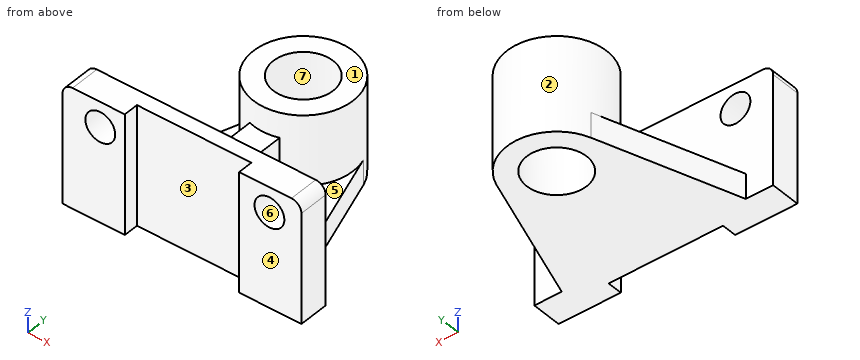
Autodesk Inventor part; units mm, degrees
ref_plane "YZ Plane" through (0, 0, 0) normal (1, 0, 0) x (0, 1, 0)
ref_plane "XZ Plane" through (0, 0, 0) normal (0, 1, 0) x (-1, 0, 0)
ref_plane "XY Plane" through (0, 0, 0) normal (0, 0, 1) x (1, 0, 0)
sketch "草图1" plane through (0, 0, 0) normal (0, 1, 0) x (-1, 0, 0)
  line L0 (24, 0) -> (-24, 0)
  line L1 (-24, 0) -> (-24, 22)
  line L2 (-22, 24) -> (22, 24)
  line L3 (24, 22) -> (24, 0)
  line L4 (0, 29.295577) -> (0, -8.008859)
  arc A0 (24, 22) -> (22, 24) centre (22, 22) ccw
  arc A1 (-22, 24) -> (-24, 22) centre (-22, 22) ccw
  line L5 (28.197943, 19) -> (-37.870085, 19) construction
  circle A2 centre (16.428853, 19) radius 3
  circle A3 centre (-17.571147, 19) radius 3
  point P0 (0, 0)
  point P1 (-24, 24)
  dimension "d0" = 24
  dimension "d1" = 48
  dimension "d2" = 2
  dimension "d3" = 5
  dimension "d4" = 6
  dimension "d5" = 6
  dimension "d6" = 34
extrude "拉伸1" add sketch "草图1" along normal blind 6
sketch "草图2" plane through (0, 0, 0) normal (0, 0, 1) x (1, 0, 0)
  line L0 (22, 0) -> (-22, 0)
  line L1 (22, 0) -> (22, 6)
  line L2 (-22, 6) -> (22, 6)
  line L3 (-22, 0) -> (-22, 6)
  line L4 (11.5, -3) -> (-11.5, -3)
  line L5 (-11.5, -3) -> (-11.5, 3)
  line L6 (-11.5, 3) -> (11.5, 3)
  line L7 (11.5, 3) -> (11.5, -3)
  line L8 (11.5, -3) -> (-11.5, 3) construction
  line L9 (-11.5, -3) -> (11.5, 3) construction
  point P0 (0, 0)
  dimension "d9" = 23
  dimension "d10" = 6
extrude "拉伸2" cut sketch "草图2" along normal blind 30 contours L7 L4 L5 L0 | L0 L5 L6 L7
sketch "草图3" plane through (0, 0, 0) normal (0, 0, 1) x (1, 0, 0)
  circle A0 centre (0, 30) radius 10
  line L0 (11.5, 3) -> (11.5, 0)
  line L1 (22, 0) -> (11.5, 0)
  line L2 (22, 0) -> (22, 6)
  line L3 (-22, 6) -> (22, 6)
  line L4 (-22, 0) -> (-22, 6)
  line L5 (-11.5, 0) -> (-22, 0)
  line L6 (-11.5, 0) -> (-11.5, 3)
  line L7 (-11.5, 3) -> (11.5, 3)
  line L8 (0, -6.997144) -> (0, 46.686565)
  circle A1 centre (0, 30) radius 6
  point P0 (0, 0)
  dimension "d13" = 20
  dimension "d14" = 30
  dimension "d15" = 12
extrude "拉伸3" add sketch "草图3" along normal blind 19 contours A0 L8 A1 | L8 A1 A0
sketch "草图4" plane through (0, 30, 0) normal (0, 0, -1) x (-1, 0, 0)
  circle A0 centre (0, 0) radius 10
  line L0 (-11.5, -30) -> (-11.5, -27)
  line L1 (-11.5, -27) -> (11.5, -27)
  line L2 (11.5, -27) -> (11.5, -30)
  line L3 (24, -30) -> (11.5, -30)
  line L4 (24, -30) -> (24, -24)
  line L5 (-24, -24) -> (24, -24)
  line L6 (-24, -30) -> (-24, -24)
  line L7 (-11.5, -30) -> (-24, -30)
  line L8 (-9.4744, 3.199335) -> (-18.5, -24)
  line L9 (9.4744, 3.199335) -> (18.5, -24)
  line L10 (0, -31.113393) -> (0, 9.909735)
  point P0 (0, -30)
  dimension "d18" = 37
sketch "草图4 outline for 拉伸4" plane through (0, 30, 0) normal (0, 0, -1) x (-1, 0, 0)
  line L0 (18.5, -24) -> (9.4744, 3.199335)
  line L1 (-18.5, -24) -> (18.5, -24)
  line L2 (-9.4744, 3.199335) -> (-18.5, -24)
  arc A0 (-9.4744, 3.199335) -> (9.4744, 3.199335) centre (0, 0) ccw
extrude "拉伸4" add sketch "草图4 outline for 拉伸4" against normal blind 5
sketch "草图5" plane through (0, 30, 5) normal (0, 0, 1) x (1, 0, 0)
  arc A0 (-9.507538, 3.099472) -> (9.507538, 3.099472) centre (0, 0) ccw
  line L0 (18.5, -24) -> (-18.5, -24)
  line L1 (3, -8) -> (-3, -8)
  line L2 (-3, -8) -> (-3, -24)
  line L3 (-3, -24) -> (3, -24)
  line L4 (3, -24) -> (3, -8)
  line L5 (3, -8) -> (-3, -24) construction
  line L6 (-3, -8) -> (3, -24) construction
  line L7 (0, -30) -> (0, 0)
  point P0 (0, -16)
  point P1 (0, -16)
  dimension "d21" = 16
  dimension "d22" = 6
extrude "拉伸5" add sketch "草图5" along normal blind 9
Verification items for the finished model (mm, model axes). Face numbers are marked on the shaded views. A direction names the side the tool comes from. Coordinates: 2 decimals unless noted, no trailing zeros. Order: outer loops, then holes, each group sorted by start corner. A loop starts at its lowest first (then second) coordinate and runs counter-clockwise, first axis right, second up. Notation, with made-up numbers: (89.5, 31) -> (123.5, 31) arc R16 ccw to (123.5, 51) -> close; hole circle Ø9 at (61, 40). An arc over 180 degrees is marked (long way). Put each result on its own line as item: value. Start each with the question number.
1) Tool access check on the marked faces 1, 2 and 3. Record the directions out of +Z, -Z, +X, -X, +Y, -Y that give a thin tool (end or side, any length) a straight path to the whole face; none if there is none.
2) Cross-section at D-D (x = -8). Enter the section's corners in (y, z), plus the area to 3 significant figures.
3) Release check for a two-part mould opening along Y. For the marked faces 4, 5, 6 and 7 record: pulls with the +Y half, pulls with the -Y half, needs draft (parallel to the pull), parting line crosses it, or undercut.
4) Cross-section at A-A (x = 0). Enter the section's corners in (y, z), plus the area to 3 significant figures.
5) Cross-section at B-B (z = 21.25). Enter the section's corners in (x, y).
6) Go/stop test with flat-tipped pins: pin 1 (12.5 mm diameter, centred on x = -9.5, y = 22.5, fed in from +Z); pin 2 (4 mm diameter, centred on y = 34.5, z = 16, fed in from +X); pin 3 (10 mm diameter, centred on y = 14.5, z = 9.5, fed in from -X); pin 4 (5.5 mm diameter, centred on x = -16.43, z = 19, fed in from +Y). Record where each tip stops, or that it passes through.
7) Material ranges on L1, parallel to Y at x = 0, z = 8.5; L2, parallel to X at y = 30, z = 14.5; L3, parallel to Y at x = -20.5, z = 5.5, recorded low to high.
8) Cross-section at C-C (y = 27). Enter the section's corners in (x, z).
Geometry check:
1. face 1: +Z, +X, -X, +Y
1. face 2: +Z
1. face 3: +Z, -Z, -Y
2. outline: (3, 0) -> (36, 0) -> (36, 19) -> (24, 19) -> (24, 5) -> (6, 5) -> (6, 24) -> (3, 24) -> close
2. area: 390 mm^2
3. face 4: pulls with the -Y half
3. face 5: undercut
3. face 6: needs draft
3. face 7: undercut
4. outline: (3, 0) -> (24, 0) -> (24, 19) -> (20, 19) -> (20, 14) -> (6, 14) -> (6, 24) -> (3, 24) -> close; (36, 0) -> (40, 0) -> (40, 19) -> (36, 19) -> close
4. area: 420 mm^2
5. outline: (-24, 0) -> (-18.41, 0) -> (-18.41, 6) -> (-24, 6) -> close; (-14.44, 0) -> (-11.5, 0) -> (-11.5, 3) -> (11.5, 3) -> (11.5, 0) -> (15.59, 0) -> (15.59, 6) -> (-14.44, 6) -> close; (19.56, 0) -> (24, 0) -> (24, 6) -> (19.56, 6) -> close
6. pin 1: stops at z = 19
6. pin 2: stops at x = 9.68
6. pin 3: stops at x = -16.4
6. pin 4: passes through
7. L1: y = 3 to 24, 36 to 40
7. L2: x = -10 to -6, 6 to 10
7. L3: y = 0 to 6
8. outline: (-11.53, 0) -> (-5.2, 0) -> (-5.2, 19) -> (-9.54, 19) -> (-9.54, 5) -> (-11.53, 5) -> close; (5.2, 0) -> (11.53, 0) -> (11.53, 5) -> (9.54, 5) -> (9.54, 19) -> (5.2, 19) -> close
